from build123d import *

# Parameters (mm, degrees)
SKETCH_1_R          = 2.1
EXTRUDE_1_DEPTH     = 4.5
SKETCH_2_R          = 2.4
EXTRUDE_2_DEPTH     = 2
FILLET_1_R          = 1.75
CUT_EXTRUDE_START   = -2
SKETCH_3_R          = 3.1
SKETCH_3_R_2        = 2.4
CUT_EXTRUDE_1_DEPTH = 2
FILLET_3_R          = 0.5


with BuildPart() as part:
    # 스케치1 → 보스-돌출1 (new, symmetric)
    with BuildSketch(Plane.XY):
        Polygon((-5, 0), (-0.385221799, 15.795303231), (1.827127146, 16.587775404), (4, -1.531866144), (6.479836305, -7.789788004), (8.009600242, -28.520515794), (5.517735363, -29.047476782), (0, -8.554669972), (-3.992979216, -4.761945907), align=None)
        Circle(SKETCH_1_R, mode=Mode.SUBTRACT)
    extrude(amount=EXTRUDE_1_DEPTH, both=True)

    # 스케치2 → 보스-돌출2 (add)
    with BuildSketch(Plane(origin=(-4.606773657, 1.345921527, 0), x_dir=(0, 0, 1), z_dir=(-0.9598722474471307, 0.2804376375966574, 0))):
        with Locations(Location((0, 8, 0), (0, 0, 90))):
            Circle(SKETCH_2_R)
    extrude(amount=EXTRUDE_2_DEPTH)

    # 필렛1
    fillet_1_edges = [part.edges().sort_by_distance(p)[0] for p in [
        (-4.956067381, 7.282081388, 0),
    ]]
    fillet(fillet_1_edges, radius=FILLET_1_R)

    # 스케치3 → 컷-돌출1 (cut)
    with BuildSketch(Plane(origin=(-4.606773657, 1.345921527, 0), x_dir=(0, 0, 1), z_dir=(-0.9598722474471308, 0.28043763759665746, 0)).offset(CUT_EXTRUDE_START)):
        with Locations(Location((0, 8, 0), (0, 0, 270))):
            Circle(SKETCH_3_R)
        with Locations(Location((0, 8, 0), (0, 0, 270))):
            Circle(SKETCH_3_R_2, mode=Mode.SUBTRACT)
    extrude(amount=CUT_EXTRUDE_1_DEPTH, mode=Mode.SUBTRACT)

    # 필렛3
    fillet_3_edges = [part.edges().sort_by_distance(p)[0] for p in [
        (1.827127146, 16.587775404, 0),
    ]]
    fillet(fillet_3_edges, radius=FILLET_3_R)


solid = part.part
Model file for the job. Use its own axes, mm. Give positions to 0.01 mm unless a question says otherwise; leave off trailing zeros. Loops run counter-clockwise (first coordinate to the right, second up) from the corner with the lowest first, then second, coordinate; pieces in that order, holes last.
1) Pull direction Z, two halves, no side cores. Call faces 1 (the flat face through (-1.969, -6.685, 0.063)), 2 (the flat face through (2, -6, 4.5)), 3 (the cylindrical face through (-1.277, 9.128, 3.074)): +Z half, -Z half, draft (parallel to the pull), parting line (faces both ways), or undercut.
2) Saw through at B-B (y = 2.5). Write the cut outline in (x, z).
3) Saw through at A-A (y = -16.5). Write the cut outline in (x, z), plus the area to 3 significant figures.
4) Wall check: line 1 (X direction, y = -16.5, z = 0); line 2 (X direction, y = 6.5, z = -1.5). Give the ranges that are in metal, low to high.
5) Flat gauge pins, fed straight in: pin 1 Ø1.5 at (y, z) = (-12.5, 1.5) entering from +X; pin 2 Ø3 at (y, z) = (-7, -2) entering from +X; pin 3 Ø6.5 at (x, y) = (0, 0) entering from -Z; pin 4 Ø1.5 at (y, z) = (0, 0.5) entering from +X. Where does each tip first touch, or does it go through?
Answer block:
1. face 1: draft
1. face 2: +Z half
1. face 3: undercut
2. outline: (-4.27, -4.5) - (3.52, -4.5) - (3.52, 4.5) - (-4.27, 4.5) - close
3. outline: (2.14, -4.5) - (7.12, -4.5) - (7.12, 4.5) - (2.14, 4.5) - close
3. area: 44.8 mm2
4. line 1: x = 2.14 to 7.12
4. line 2: x = -1.02 to 3.04
5. pin 1: stops at x = 6.88
5. pin 2: stops at x = 6.53
5. pin 3: stops at z = -4.5
5. pin 4: stops at x = 3.91
